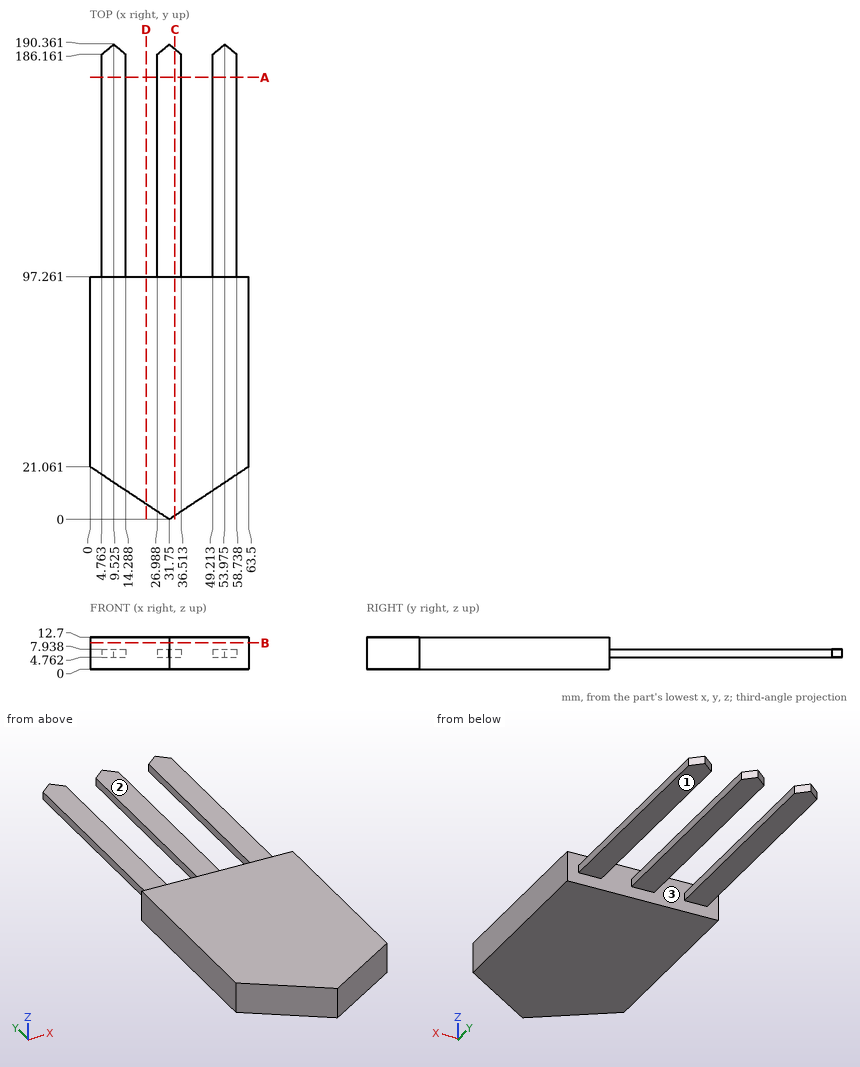
Geometry: see drawing. Coordinates: mm, zero at the bounding-box minimum. A direction names the side the tool comes from. Round coordinates to 2 decimals unless told otherwise and drop trailing zeros. Write each loop counter-clockwise with the first axis right and the second up, starting at its lowest first coordinate (ties: lowest second). Pieces come first, ordered by that corner, then holes. Notation, with made-up numbers: M -22.5,60 L 3.5,60 A13 cw 3.5,76 Z; hole C 59.25,50 d5. An arc over 180 degrees is marked long. Answer in a Markdown table with one row per item. Add a question column.
(1) Cut plane C-C, the plane x = 34. Return the cut outline in (y, z).
(2) Cut plane B-B, the plane z = 10.5. Return the cut outline in (x, y).
(3) Ray query, L1, parallel to X at y = 160, z = 7; L2, parallel to Z at x = 5, y = 128; L3, parallel to Y at x = 18.5, z = 7. Return the intervals inside material, ascending.
(4) Cut plane A-A, the plane y = 177. Return the cut outline in (x, z).
(5) Contact query for flat-ended pins moving along their axis: pin 1 (2.5 mm diameter, centred on y = 141, z = 7, fed in from +X); pin 2 (5 mm diameter, centred on x = 54.5, y = 123, fed in from +Z); pin 3 (1 mm diameter, centred on y = 125, z = 6, fed in from -X); pin 4 (1.5 mm diameter, centred on y = 144.5, z = 10, fed in from +X) (3 decimals). Output: stop coordinate, or through.
(6) Cut plane D-D, the plane x = 22.5. Return the cut outline in (y, z) (1 decimal).
(7) Reachability of the marked faces 1, 2 and 3 from +Z, -Z, +X, -X, +Y, -Y: full face, straight path, thin tool, end or side. Return the list, or none.
Established:
| question | item | result |
|---|---|---|
| 1 | outline | M 1.49,0 L 97.26,0 L 97.26,4.76 L 188.38,4.76 L 188.38,7.94 L 97.26,7.94 L 97.26,12.7 L 1.49,12.7 Z |
| 2 | outline | M 0,21.06 L 31.75,0 L 63.5,21.06 L 63.5,97.26 L 0,97.26 Z |
| 3 | L1 | 4.76 to 14.29, 26.99 to 36.51, 49.21 to 58.74 |
| 3 | L2 | 4.76 to 7.94 |
| 3 | L3 | 8.79 to 97.26 |
| 4 | outline | M 4.76,4.76 L 14.29,4.76 L 14.29,7.94 L 4.76,7.94 Z; M 26.99,4.76 L 36.51,4.76 L 36.51,7.94 L 26.99,7.94 Z; M 49.21,4.76 L 58.74,4.76 L 58.74,7.94 L 49.21,7.94 Z |
| 5 | pin 1 | x = 58.74 |
| 5 | pin 2 | z = 7.94 |
| 5 | pin 3 | x = 4.76 |
| 5 | pin 4 | through |
| 6 | outline | M 6.1,0 L 97.3,0 L 97.3,12.7 L 6.1,12.7 Z |
| 7 | face 1 | -Z, +X, -X, +Y |
| 7 | face 2 | +Z, +X, -X, +Y |
| 7 | face 3 | +Y |
